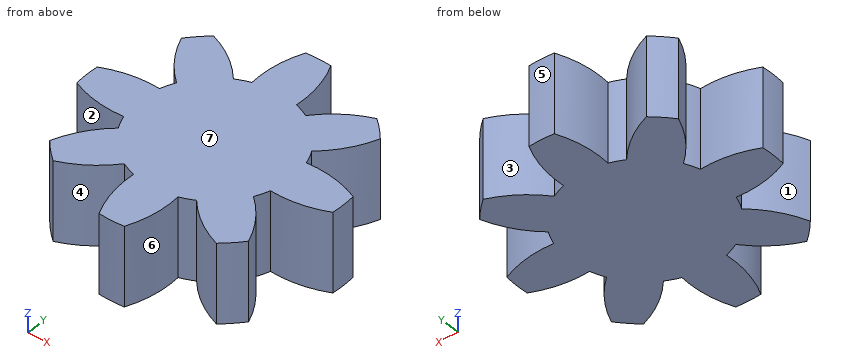
Autodesk Inventor part; units mm, degrees
ref_plane "Work Plane2" through (0, 0, 3) normal (0, 0, 1) x (1, 0, 0)
ref_plane "Work Plane8" through (0, 0, 0) normal (0.9238795, 0.3826834, 0) x (0, 0, 1)
ref_plane "Work Plane9" through (0, 0, 0) normal (1, 0, 0) x (0, 1, 0)
sketch "Sketch1" plane through (0, 0, 0) normal (0, 0, 1) x (1, 0, 0)
  circle A0 centre (0, 0) radius 9.575
  dimension "d0" = 19.15
extrude "Extrusion1" add sketch "Sketch1" along normal blind 6
ref_plane "Work Plane2" through (0, 0, 3) normal (0, 0, 1) x (1, 0, 0)
sketch "Sketch2" plane through (0, 0, 0) normal (0, 0, -1) x (-1, 0, 0)
  circle A0 centre (0, 0) radius 9.575
  circle A1 centre (0, 0) radius 7
  dimension "d3" = 14
surface extrude "Pitch Diameter" sketch "Sketch2" against normal through all shown no curves A1
ref_plane "Work Plane8" through (0, 0, 0) normal (0.9238795, 0.3826834, 0) x (0, 0, 1)
ref_plane "Work Plane9" through (0, 0, 0) normal (1, 0, 0) x (0, 1, 0)
spur gear teeth "Spur Gear" teeth 8 pitch diameter 14 tip diameter 19.15 root diameter 11.408 face width 20 start plane through (0, 0, 0) normal (0, 0, -1) x (-1, 0, 0)
equation "\"d0\" = da_da"
equation "\"d3\" = da_d"
equation "\"d16\" = da_aw"
equation "\"d43\" = da_aw"
equation "\"d46\" = da_aw"
properties part number "Spur Gear2" material "Steel"
Here's how the part is built. I have some questions about the finished solid (model axes, mm). Face numbers are marked on the shaded views. A direction names the side the tool comes from. Coordinates: 2 decimals unless noted, no trailing zeros. Write each loop counter-clockwise with the first axis right and the second up, starting at its lowest first coordinate (ties: lowest second). Pieces come first, ordered by that corner, then holes.
Item 1: I want a section at A-A on y = -7. Write out the boundary of the cut face in (x, z), and give its area (3 significant figures).
Item 2: If I drill on line 1 (X direction, y = -5.75, z = 1.35); line 2 (Y direction, x = -6.75, z = 2.45); line 3 (Y direction, x = 6.5, z = 4.45), over which ranges is the centre line in solid material (lowest first)?
Item 3: On a 3-axis mill with a long thin cutter (end or side, diameter ignored), from which of +Z, -Z, +X, -X, +Y, -Y can I reach the whole of each face in a straight line? I mean the marked faces 1, 2, 3 and 4. Say none if no direction works.
Item 4: I want a section at D-D on x = 3.25. Write out the boundary of the cut face in (y, z), and give its area (3 significant figures).
Item 5: If we mould it in two halves opening along X, with no side actions, what happens to the marked faces 5, 6 and 7? For each: +X half, -X half, draft (parallel to the pull), parting line (faces both ways), or undercut.
Findings below:
1. outline: (-6.53, 0) - (-5.16, 0) - (-5.16, 6) - (-6.53, 6) - close; (-1.64, 0) - (1.64, 0) - (1.64, 6) - (-1.64, 6) - close; (5.16, 0) - (6.53, 0) - (6.53, 6) - (5.16, 6) - close
1. area: 36.2 mm2
2. line 1: x = -7.27 to -3.38, -1.68 to 1.68, 3.38 to 7.27
2. line 2: y = -6.79 to -4.71, -1.66 to 1.66, 4.71 to 6.79
2. line 3: y = -7.03 to -4.32, -1.68 to 1.68, 4.32 to 7.03
3. face 1: +Z, -Z, -X
3. face 2: +Z, -Z
3. face 3: +Z, -Z, +Y
3. face 4: +Z, -Z, -Y
4. outline: (-5.63, 0) - (5.63, 0) - (5.63, 6) - (-5.63, 6) - close
4. area: 67.6 mm2
5. face 5: parting line
5. face 6: undercut
5. face 7: draft
